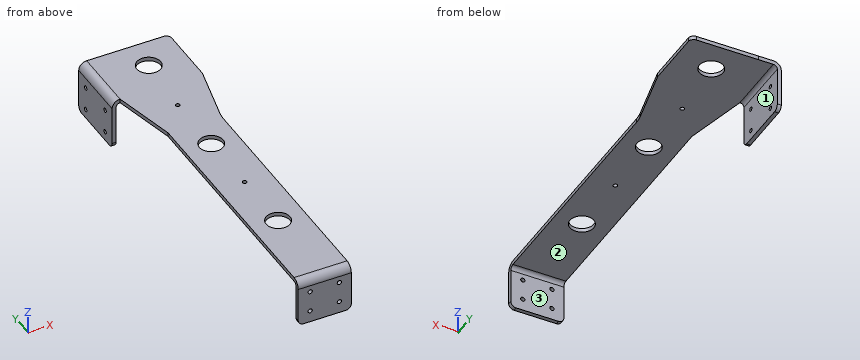
Autodesk Inventor part; units mm, degrees
ref_plane "YZ Plane" through (0, 0, 0) normal (1, 0, 0) x (0, 1, 0)
ref_plane "XZ Plane" through (0, 0, 0) normal (0, 1, 0) x (-1, 0, 0)
ref_plane "XY Plane" through (0, 0, 0) normal (0, 0, 1) x (1, 0, 0)
sketch "Sketch1" plane through (0, 0, 0) normal (0, 0, 1) x (1, 0, 0)
  line L0 (31.75, -148.4313) -> (-31.75, -148.4313)
  line L1 (-31.75, -148.4313) -> (-31.75, 148.4313)
  line L2 (-31.75, 148.4313) -> (31.75, 148.4313) construction
  line L3 (31.75, 148.4313) -> (31.75, -148.4313)
  line L4 (31.75, -148.4313) -> (-31.75, 148.4313) construction
  line L5 (-31.75, -148.4313) -> (31.75, 148.4313) construction
  line L6 (31.75, 148.4313) -> (49.2125, 224.6313)
  line L7 (-31.75, 148.4313) -> (-31.75, 300.8312) construction
  line L8 (-31.75, 300.8312) -> (49.2125, 300.8313)
  line L9 (49.2125, 224.6313) -> (49.2125, 300.8313)
  line L10 (-31.75, 300.8312) -> (-49.2125, 300.8312)
  line L11 (-49.2125, 300.8312) -> (-49.2125, 224.6312)
  line L12 (-49.2125, 224.6312) -> (-31.75, 224.6312) construction
  line L13 (-31.75, 224.6312) -> (-31.75, 300.8312) construction
  line L14 (-49.2125, 224.6312) -> (-31.75, 148.4313)
  point P0 (0, 0)
  dimension "d0" = 63.5
  dimension "d1" = 296.8625
  dimension "d2" = 80.9625
  dimension "d3" = 152.4
  dimension "d43" = 76.2
  dimension "d63" = 17.4625
  dimension "d64" = 76.2
extrude "Plate1" add sketch "Sketch1" along normal blind 4.7625
sketch "Sketch2" plane through (0, 0, 4.7625) normal (0, 0, 1) x (1, 0, 0)
  line L0 (31.75, -148.4313) -> (-31.75, -148.4313) construction
  line L1 (-31.75, -148.4313) -> (-31.75, 148.4313) construction
  line L2 (0, 110.5852) -> (5.3275, 263.1463) construction
  line L3 (0, 110.5852) -> (152.654, 110.5852) construction
  point P0 (0, 0)
  point P1 (0, -42.0688)
  point P2 (0, -148.4313)
  point P3 (-31.75, 300.0375)
  dimension "d5" = 106.3625
  dimension "d8" = 152.654
  dimension "d29" = 31.75
  dimension "d98" = 152.654
  dimension "d99" = 88
hole "Hole1" at (0, 110.5852, 4.7625) at (5.3275, 263.1463, 4.7625) at (0, -42.0688, 4.7625) direction (0, 0, -1) diameter 28.575 end through all
sketch "Sketch3" plane through (0, 0, 4.7625) normal (0, 0, 1) x (1, 0, 0)
  circle A0 centre (0, 110.5852) radius 14.2875 construction
  line L0 (0, 110.5852) -> (0, -42.0688) construction
  line L1 (0, 110.5852) -> (0, 263.2392) construction
  circle A1 centre (5.3275, 262.3525) radius 14.2875
  circle A2 centre (0, -42.8625) radius 14.2875
  point P0 (0, 0)
  point P1 (0, 186.9122)
  point P2 (0, 34.2582)
hole "Hole2" at (0, 34.2582, 4.7625) at (0, 186.9122, 4.7625) direction (0, 0, -1) diameter 5.1054 end through all
fillet "Corner Round1" radius 50.8 1 edges at (31.75, 148.4313, 2.3813)
sketch "Sketch5" plane through (-31.75, -143.6687, 4.7625) normal (0, -1, 0) x (1, 0, 0)
  line L0 (63.5, 0) -> (0, 0)
  line L1 (0, 0) -> (0, -57.15)
  line L2 (0, -57.15) -> (63.5, -57.15)
  line L3 (63.5, -57.15) -> (63.5, 0)
edge flange "Flange2" height 52.3875 angle 90 thickness 4.7625 bend radius 4.7625 thickness toward (0, -1, 0) relief tear relief width 4.7625 relief depth 2.3813 edges at (0, -148.4313, 0) wall of the first edge with corners at (31.75, -143.6687, 4.7625) (-31.75, -143.6687, 4.7625) (-31.75, -143.6687, -52.3875) (31.75, -143.6687, -52.3875)
bend "Bend2"
corner "Corner2"
sketch "Sketch7" plane through (-53.975, 300.8312, -4.7625) normal (-1, 0, 0) x (0, -1, 0)
  line L0 (76.2, 0) -> (0, 0)
  line L1 (0, 0) -> (0, -52.3875)
  line L2 (0, -52.3875) -> (76.2, -52.3875)
  line L3 (76.2, -52.3875) -> (76.2, 0)
edge flange "Flange3" height 61.9125 angle 90 thickness 4.7625 bend radius 4.7625 thickness toward (-1, 0, 0) relief tear relief width 4.7625 relief depth 2.3813 edges at (-49.2125, 262.7312, 0) wall of the first edge with corners at (-53.975, 224.6312, -4.7625) (-53.975, 300.8312, -4.7625) (-53.975, 300.8312, -57.15) (-53.975, 224.6312, -57.15)
bend "Bend3"
corner "Corner3"
sketch "Sketch8" plane through (-58.7375, 224.6312, -57.15) normal (-1, 0, 0) x (0, 0, 1)
  line L0 (0, 76.2) -> (52.3875, 76.2)
  line L1 (0, 0) -> (0, 76.2)
  line L2 (52.3875, 0) -> (52.3875, 76.2) construction
  point P0 (57.15, -224.6312)
  point P1 (39.6875, 60.325)
  point P2 (39.6875, 15.875)
  point P3 (11.1125, 15.875)
  point P4 (11.1125, 60.325)
  dimension "d75" = 44.45
  dimension "d76" = 28.575
  dimension "d77" = 15.875
  dimension "d101" = 12.7
hole "Hole4" at (-58.7375, 284.9562, -17.4625) at (-58.7375, 240.5062, -17.4625) at (-58.7375, 240.5062, -46.0375) at (-58.7375, 284.9562, -46.0375) direction (1, 0, 0) diameter 5.1054 end through all
sketch "Sketch9" plane through (-31.75, -148.4313, -52.3875) normal (0, -1, 0) x (1, 0, 0)
  line L0 (0, 0) -> (0, 47.625)
  line L1 (0, 57.15) -> (63.5, 57.15)
  line L2 (63.5, 0) -> (0, 0)
  point P0 (31.75, 52.3875)
  point P1 (14.2875, 39.6875)
  point P2 (49.2125, 39.6875)
  point P3 (49.2125, 14.2875)
  point P4 (14.2875, 14.2875)
  dimension "d86" = 14.2875
  dimension "d87" = 25.4
  dimension "d88" = 34.925
  dimension "d90" = 14.2875
hole "Hole5" at (-17.4625, -148.4313, -12.7) at (17.4625, -148.4313, -12.7) at (17.4625, -148.4313, -38.1) at (-17.4625, -148.4313, -38.1) direction (0, 1, 0) diameter 5.1054 end through all
fillet "Corner Round2" radius 6.35 5 edges at (-56.3563, 224.6312, -57.15) (-56.3563, 300.8312, -57.15) (-31.75, -146.05, -52.3875) (31.75, -146.05, -52.3875) (49.2125, 300.8313, 2.3813)
equation "\"d18\" = Thickness"
equation "\"d84\" = Thickness"
equation "\"d4\" = Thickness"
equation "\"d44\" = BendReliefWidth"
equation "\"d45\" = BendReliefDepth"
equation "\"d46\" = MinimumRemnant"
equation "\"d47\" = TransitionRadius"
equation "\"d50\" = BendRadius"
equation "\"d51\" = CornerReliefSize"
equation "\"d52\" = GapSize"
equation "\"d53\" = JacobiRadiusSize"
equation "\"d65\" = BendReliefWidth"
equation "\"d66\" = BendReliefDepth"
equation "\"d67\" = MinimumRemnant"
equation "\"d68\" = TransitionRadius"
equation "\"d71\" = BendRadius"
equation "\"d72\" = CornerReliefSize"
equation "\"d73\" = GapSize"
equation "\"d74\" = JacobiRadiusSize"
equation "\"BendRadius\" = Thickness"
equation "\"BendReliefWidth\" = Thickness"
equation "\"BendReliefDepth\" = 0.5 * Thickness"
equation "\"CornerReliefSize\" = 4 * Thickness"
equation "\"MinimumRemnant\" = 2 * Thickness"
equation "\"TransitionRadius\" = BendRadius"
equation "\"JacobiRadiusSize\" = BendRadius"
equation "\"GapSize\" = Thickness"
properties part number "feeder_guide_plate" material "Polycarbonate, Clear"
Check sheet for the modelled part. Datum: model origin and axes. Units: mm. Face numbers are marked on the shaded views. A direction names the side the tool comes from. Give positions to 0.01 mm unless a question says otherwise; leave off trailing zeros. Loops run counter-clockwise (first coordinate to the right, second up) from the corner with the lowest first, then second, coordinate; pieces in that order, holes last. Notation, with made-up numbers: M 32.25,49.5 L 90.25,49.5 A34 cw 90.25,79.5 Z; hole C 65.5,34.25 d3. An arc over 180 degrees is marked long. Use a Markdown table: item, result. Add a question column.
Q1. Scan lines: line 1 along X through (y, z) = (-144.95, -38.1); line 2 along Z through (x, y) = (-8, 90.5); line 3 along Y through (x, z) = (0, 3.45). Record each from-to range of solid material in increasing order. Write a range as [from, to].
Q2. Tool access check on the marked faces 1, 2 and 3. Record the directions out of +Z, -Z, +X, -X, +Y, -Y that give a thin tool (end or side, any length) a straight path to the whole face; none if there is none.
Q3. Go/stop test with flat-tipped pins: pin 1 (12 mm diameter, centred on x = -26, z = -13, fed in from +Y); pin 2 (10.5 mm diameter, centred on x = -53, z = -28, fed in from -Y); pin 3 (4 mm diameter, centred on y = 284.96, z = -46.04, fed in from +X); pin 4 (8 mm diameter, centred on y = 240.51, z = -17.46, fed in from +X) (3 decimals). Record where each tip stops, or that it passes through.
Q4. Sectioned sample at A-A, the plane y = -64. Record the cut outline in (x, z), then the cut area to 3 significant figures.
Q5. Sectioned sample at B-B, the plane y = 219. Record the cut outline in (x, z).
Verdict:
| question | item | result |
|---|---|---|
| 1 | line 1 | [-31.75, -20.02], [-14.91, 14.91], [20.02, 31.75] |
| 1 | line 2 | [0, 4.76] |
| 1 | line 3 | [-143.73, -56.36], [-27.78, 31.71], [36.81, 96.3], [124.87, 184.36], [189.46, 249.89], [276.4, 300.83] |
| 2 | face 1 | -Z, +X, +Y, -Y |
| 2 | face 2 | -Z, +X, +Y |
| 2 | face 3 | -Z, +X, -X, +Y |
| 3 | pin 1 | y = -143.67 |
| 3 | pin 2 | y = 224.63 |
| 3 | pin 3 | through |
| 3 | pin 4 | x = -53.975 |
| 4 | outline | M -31.75,0 L 31.75,0 L 31.75,4.76 L -31.75,4.76 Z |
| 4 | area | 302 mm^2 |
| 5 | outline | M -47.92,0 L 47.92,0 L 47.92,4.76 L -47.92,4.76 Z |
